The figure shows three views and two pictorial views of one solid part (mm, origin at its lowest corner). Answer the questions. A direction names the side the tool comes from. Coordinates: 2 decimals unless noted, no trailing zeros. Write each loop counter-clockwise with the first axis right and the second up, starting at its lowest first coordinate (ties: lowest second). Pieces come first, ordered by that corner, then holes. Notation, with made-up numbers: M 29.5,83 L 80.5,83 A15 ccw 80.5,112 Z; hole C -20,18 d1. An arc over 180 degrees is marked long. Write item = value, one per line.
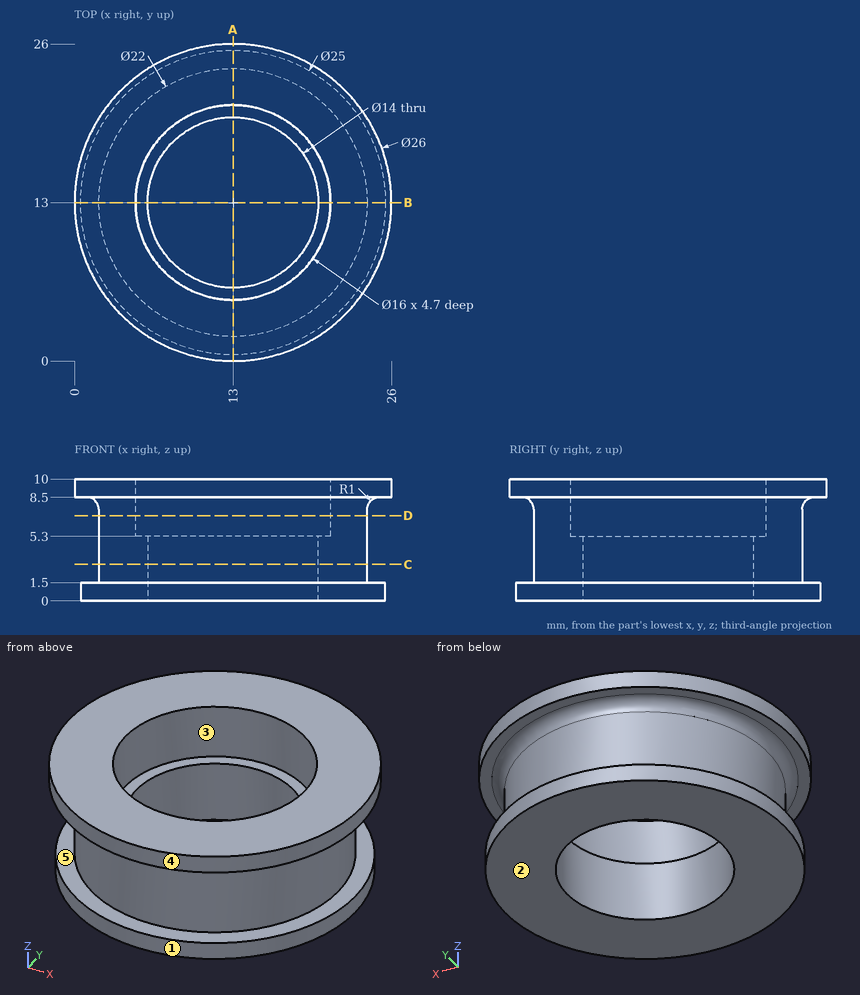
Item 1: For a pull along X with two mould halves and no side action, classify the marked faces 1, 2 and 3 as released by +X, released by -X, zero draft, split by the parting line, or undercut.
Worked answers:
face_1 = split by the parting line
face_2 = zero draft
face_3 = undercut
Item 2: Find section A-A (x = 13). Determine the outline of the cut face in (y, z).
Worked answers:
outline = M 0,8.5 L 1,8.5 A1 cw 2,7.5 L 2,1.5 L 0.5,1.5 L 0.5,0 L 6,0 L 6,5.3 L 5,5.3 L 5,10 L 0,10 Z; M 20,0 L 25.5,0 L 25.5,1.5 L 24,1.5 L 24,7.5 A1 cw 25,8.5 L 26,8.5 L 26,10 L 21,10 L 21,5.3 L 20,5.3 Z
Item 3: Consider line 1 along Y through (x, z) = (13, 6.7); line 2 along X through (y, z) = (13, 2.45); line 3 along X through (y, z) = (13, 8.55). Determine where each line is inside the solid, lowest interval first. Write a range as from..to.
Worked answers:
line_1 = 2..5, 21..24
line_2 = 2..6, 20..24
line_3 = 0..5, 21..26
Item 4: Find section D-D (z = 7). Determine the outline of the cut face in (x, y), and give its area (3 significant figures).
Worked answers:
outline = C 13,13 d22; hole C 13,13 d16
area = 179 mm²
Item 5: Flat-ended cylindrical pins translate along their axes: pin 1 (3 mm diameter, centred on x = 9.5, z = 4.5, fed in from -Y); pin 2 (6 mm diameter, centred on y = 8, z = 2.5, fed in from -X); pin 3 (3 mm diameter, centred on x = 18.5, z = 1.5, fed in from -Y); pin 4 (12.5 mm diameter, centred on x = 13, y = 13, fed in from +Z). Find the tip coordinate at first contact, or state that the pin passes through.
Worked answers:
pin_1 = 2.18
pin_2 = 0.69
pin_3 = 1.16
pin_4 = through
Item 6: Which of the six approach directions +Z, -Z, +X, -X, +Y, -Y give full straight-line access (tool end or side, diameter ignored) to the marked faces 4 and 5?
Worked answers:
face_4 = +Z, -Z
face_5 = none
Item 7: Find section C-C (z = 3). Determine the outline of the cut face in (x, y).
Worked answers:
outline = C 13,13 d22; hole C 13,13 d14
